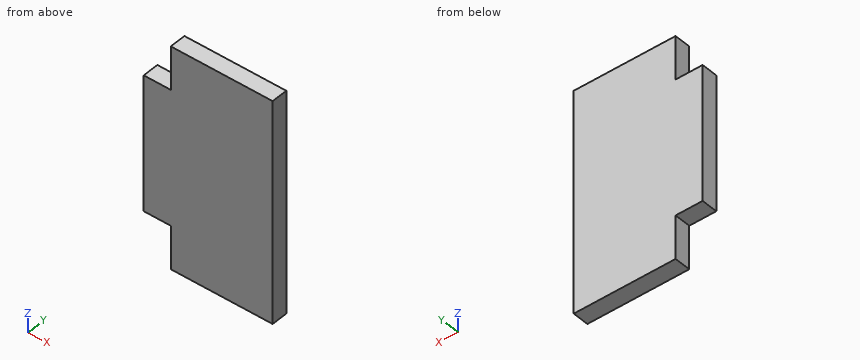
Autodesk Inventor part; units mm, degrees
ref_plane "YZ Plane" through (0, 0, 0) normal (1, 0, 0) x (0, 1, 0)
ref_plane "XZ Plane" through (0, 0, 0) normal (0, 1, 0) x (-1, 0, 0)
ref_plane "XY Plane" through (0, 0, 0) normal (0, 0, 1) x (1, 0, 0)
sketch "Sketch1" plane through (0, 0, 0) normal (0, 1, 0) x (-1, 0, 0)
  line L0 (-42.845, -43.5625) -> (-42.845, 65.5625)
  line L1 (33.4911, -43.5625) -> (33.4911, 65.5625)
  line L2 (33.4911, 30) -> (33.4911, -8)
  line L3 (-42.845, -8) -> (-42.845, 30)
  line L4 (-42.845, -43.5625) -> (-42.845, 65.5625)
  line L5 (-42.845, 30) -> (-17.845, 30)
  line L6 (-17.845, 30) -> (-17.845, -8)
  line L7 (-17.845, -8) -> (-42.845, -8)
  line L8 (-42.845, -8) -> (-42.845, 30)
  line L9 (33.4911, 30) -> (8.4911, 30)
  line L10 (8.4911, 30) -> (8.4911, -8)
  line L11 (8.4911, -8) -> (33.4911, -8)
  line L12 (33.4911, -8) -> (33.4911, 30)
  line L13 (-17.845, 30) -> (-17.845, -8)
  line L14 (8.4911, -8) -> (8.4911, 30)
  line L15 (-17.845, 30) -> (-15.845, 30)
  line L16 (-15.845, 30) -> (-15.845, -8)
  line L17 (-15.845, -8) -> (-17.845, -8)
  line L18 (-17.845, -8) -> (-17.845, 30)
  line L19 (8.4911, 30) -> (6.4911, 30)
  line L20 (6.4911, 30) -> (6.4911, -8)
  line L21 (6.4911, -8) -> (8.4911, -8)
  line L22 (8.4911, -8) -> (8.4911, 30)
  line L23 (-15.845, -8) -> (-15.845, 30)
  line L24 (6.4911, 30) -> (6.4911, -8)
  line L25 (-15.845, -8) -> (-15.845, 30)
  line L26 (-15.845, 30) -> (-15.845, -8)
  line L27 (0, 22) -> (0, 40.5625)
  line L28 (-17.845, -8) -> (0, -8)
  line L29 (0, -8) -> (0, 30)
  line L30 (0, 30) -> (-17.845, 30)
  line L31 (-17.845, 30) -> (-17.845, -8)
  line L32 (5, 22) -> (5, 0)
  line L33 (0, 22) -> (5, 22)
  line L34 (5, 22) -> (5, 0)
  line L35 (5, 0) -> (0, 0)
  line L36 (0, 0) -> (0, 22)
  line L37 (1.5, 31.5) -> (-17.345, 31.5)
  line L38 (-17.345, 31.5) -> (-17.345, -9.5)
  line L39 (-17.345, -9.5) -> (1.5, -9.5)
  line L40 (1.5, -9.5) -> (1.5, 31.5)
  line L41 (6.5, 23.5) -> (0, 23.5)
  line L42 (0, 23.5) -> (0, -1.5)
  line L43 (0, -1.5) -> (6.5, -1.5)
  line L44 (6.5, -1.5) -> (6.5, 23.5)
  point P0 (-45.9471, 11)
  point P1 (-45.845, 65.5625)
  point P2 (36.4911, 65.5625)
  point P3 (-42.845, 11)
  point P4 (-42.845, 11)
  dimension "d0" = 38
  dimension "d1" = 25
  dimension "d2" = 38
  dimension "d3" = 25
  dimension "d4" = 2
  dimension "d5" = 2
  dimension "d6" = 1.5
  dimension "d7" = 1.5
  dimension "d8" = 1.5
  dimension "d9" = 1.5
  dimension "d10" = 1.5
  dimension "d11" = 1.5
  dimension "d12" = 1.5
extrude "Extrusion1" add sketch "Sketch1" along normal blind 3 contours L38 L15 L16 L17 | L17 L28 L29 L43 L40 L39 L38 | L38 L37 L27 L30 L15 | L16 L30 L27 L29 L28 | L27 L37 L40 L41 | L29 L35 L40 L43 | L40 L35 L32 L33 L41 L20 L43 | L41 L40 L33 L27 | L29 L33 L40 L35 | L40 L33 L32 L35 | L20 L41 L44 L43
equation "\"d8\" = d7"
equation "\"d9\" = d7"
equation "\"d10\" = d9"
equation "\"d11\" = d7"
equation "\"d12\" = d7"
properties part number "bottom perspex"
Input: part model. Units: mm. Frame: model coordinates. Give positions to 0.01 mm unless a question says otherwise; leave off trailing zeros. Order: outer loops, then holes, each group sorted by start corner. A loop starts at its lowest first (then second) coordinate and runs counter-clockwise, first axis right, second up. Notation, with made-up numbers: M -30.5,-16.5 L -10.5,-16.5 A24 ccw -10.5,-1.5 Z; hole C -34,3 d4. An arc over 180 degrees is marked long. Return JSON: item names as keys, results as strings.
1) Line query: L1, parallel to Z at x = -3, y = 1.15; L2, parallel to X at y = 2.8, z = -2 (3 decimals). Output: solid intervals per line, ascending. Write a range as [from, to].
Taken from the geometry:
{"L1": "z = [-1.5, 23.5]", "L2": "x = [-1.5, 17.345]"}
2) Section query B-B on z = 29.5. Output: boundary loops of the cut face in (x, y) (3 decimals), and give its area (3 significant figures).
Taken from the geometry:
{"outline": "M -1.5,0 L 17.345,0 L 17.345,3 L -1.5,3 Z", "area": "56.5 mm2"}
3) Section query A-A on y = 1.7. Output: boundary loops of the cut face in (x, z) (3 decimals).
Taken from the geometry:
{"outline": "M -6.5,-1.5 L -1.5,-1.5 L -1.5,-9.5 L 17.345,-9.5 L 17.345,31.5 L -1.5,31.5 L -1.5,23.5 L -6.5,23.5 Z"}
4) Contact query for flat-ended pins moving along their axis: pin 1 (1.5 mm diameter, centred on y = 1.5, z = 29, fed in from -X); pin 2 (0.9 mm diameter, centred on x = -5, y = 1, fed in from +Z). Output: stop coordinate, or through.
Taken from the geometry:
{"pin 1": "stops at x = -1.5", "pin 2": "stops at z = 23.5"}
